Input: part model. Units: mm. Frame: model coordinates. A direction names the side the tool comes from. Coordinates: 2 decimals unless noted, no trailing zeros. Order: outer loops, then holes, each group sorted by start corner. A loop starts at its lowest first (then second) coordinate and runs counter-clockwise, first axis right, second up. Notation, with made-up numbers: M 1,-3.75 L 49,-3.75 A32 cw 49,25.25 Z; hole C 11.25,-39 d10. An arc over 180 degrees is marked long. Answer in a Markdown table with one row per item.
from build123d import *

# Parameters (mm, degrees)
SKETCH1_R                    = 4.25
BASE_FLANGE1_DEPTH           = 3.175
EDGE_FLANGE1_DEPTH           = 20
EDGE_FLANGE1_START           = 3.175
EDGE_FLANGE1_FLAT_DEPTH      = 3.175
EDGE_FLANGE3_STRIP_W         = 15.24
EDGE_FLANGE3_STRIP_H         = 3.175
EDGE_FLANGE3_STRIP_CUT_DEPTH = 20
EDGE_FLANGE3_DEPTH           = 20
EDGE_FLANGE3_START           = -3.175
EDGE_FLANGE3_PROFILE_R       = 4.25
EDGE_FLANGE3_FLAT_DEPTH      = 3.175


# Sheet-metal steps are written as plain solids
with BuildPart() as part:
    # Sketch1 → Base-Flange1 (new body)
    with BuildSketch(Plane.XY):
        with BuildLine():
            Line((12.5, 10), (0, 10))
            ThreePointArc((0, 10), (-10, 0), (0, -10))
            Line((0, -10), (12.5, -10))
            Line((12.5, -10), (12.5, 10))
        make_face()
        Circle(SKETCH1_R, mode=Mode.SUBTRACT)
    extrude(amount=-BASE_FLANGE1_DEPTH)

    # Edge-Flange1 bend section (across the edge) → Edge-Flange1 (add)
    with BuildSketch(Plane(origin=(13.77, -10, 0), x_dir=(-1, 0, 0), z_dir=(0, 1, 0))):
        with BuildLine():
            Line((-3.175, 1.27), (0, 1.27))
            ThreePointArc((0, 1.27), (0.371974388, 0.371974388), (1.27, 0))
            Line((1.27, 0), (1.27, -3.175))
            ThreePointArc((1.27, -3.175), (-1.873089642, -1.873089642), (-3.175, 1.27))
        make_face()
    extrude(amount=EDGE_FLANGE1_DEPTH)

    # Edge-Flange1 profile (on flange) → Edge-Flange1 flat (add)
    with BuildSketch(Plane.YZ.offset(13.77).offset(EDGE_FLANGE1_START)):
        with BuildLine():
            Line((36.2752, 26.825), (5, 26.825))
            ThreePointArc((5, 26.825), (-5.606601718, 22.431601718), (-10, 11.825))
            Line((-10, 11.825), (-10, 1.27))
            Line((-10, 1.27), (10, 1.27))
            Line((10, 1.27), (10, 1.825))
            ThreePointArc((10, 1.825), (11.464466094, 5.360533906), (15, 6.825))
            Line((15, 6.825), (36.2752, 6.825))
            Line((36.2752, 6.825), (36.2752, 26.825))
        make_face()
    extrude(amount=-EDGE_FLANGE1_FLAT_DEPTH)

    # Edge-Flange3 strip (across the edge) → Edge-Flange3 strip cut (cut)
    with BuildSketch(Plane(origin=(16.945, 36.2752, 6.825), x_dir=(0, -1, 0), z_dir=(0, 0, 1))):
        with Locations((-6.35, -1.5875)):
            Rectangle(EDGE_FLANGE3_STRIP_W, EDGE_FLANGE3_STRIP_H)
    extrude(amount=EDGE_FLANGE3_STRIP_CUT_DEPTH, mode=Mode.SUBTRACT)

    # Edge-Flange3 bend section (across the edge) → Edge-Flange3 (add)
    with BuildSketch(Plane(origin=(16.945, 36.2752, 6.825), x_dir=(0, -1, 0), z_dir=(0, 0, 1))):
        with BuildLine():
            Line((-3.175, 1.27), (0, 1.27))
            ThreePointArc((0, 1.27), (0.371974388, 0.371974388), (1.27, 0))
            Line((1.27, 0), (1.27, -3.175))
            ThreePointArc((1.27, -3.175), (-1.873089642, -1.873089642), (-3.175, 1.27))
        make_face()
    extrude(amount=EDGE_FLANGE3_DEPTH)

    # Edge-Flange3 profile (on flange) → Edge-Flange3 flat (add)
    with BuildSketch(Plane(origin=(16.945, 36.2752, 0), x_dir=(0, 0, -1), z_dir=(0, -1, 0)).offset(EDGE_FLANGE3_START)):
        with BuildLine():
            ThreePointArc((-6.825, 3.0675), (-14.14733047, 20.74516953), (-31.825, 28.0675))
            Line((-31.825, 28.0675), (-70.925400974, 28.0675))
            ThreePointArc((-70.925400974, 28.0675), (-79.925400974, 19.0675), (-70.925400974, 10.0675))
            Line((-70.925400974, 10.0675), (-31.825, 10.0675))
            ThreePointArc((-31.825, 10.0675), (-28.289466094, 8.603033906), (-26.825, 5.0675))
            Line((-26.825, 5.0675), (-26.825, 1.27))
            Line((-26.825, 1.27), (-6.825, 1.27))
            Line((-6.825, 1.27), (-6.825, 3.0675))
        make_face()
        with Locations((-70.925400974, 19.0675)):
            Circle(EDGE_FLANGE3_PROFILE_R, mode=Mode.SUBTRACT)
    extrude(amount=EDGE_FLANGE3_FLAT_DEPTH)


solid = part.part
1) Reachability of faces 1 (the face through (15, 27, 6.825)), 2 (the face through (35, 36.275, 44)), 3 (the face through (36.21, 37.885, 79.923)), 4 (the face through (13.77, 12, 14)) from +Z, -Z, +X, -X, +Y, -Y: full face, straight path, thin tool, end or side. Return the list, or none.
Resolved:
| item | result |
|---|---|
| face 1 | -Z, +X, -X, +Y |
| face 2 | +Z, -Z, +X, -Y |
| face 3 | +Z, +Y, -Y |
| face 4 | +Z, -X, +Y, -Y |
2) Material intervals for probe 1 along Y at (x, z) = (0, -1.7); probe 2 along Z at (x, y) = (6, 7.5) (3 decimals); probe 3 along X at (y, z) = (3, 11) (3 decimals), sorted ascending.
Resolved:
| item | result |
|---|---|
| probe 1 | y = -10 to -4.25, 4.25 to 10 |
| probe 2 | z = -3.175 to 0 |
| probe 3 | x = 13.77 to 16.945 |
3) Contact query for flat-ended pins moving along their axis: pin 1 (13.5 mm diameter, centred on x = 36.01, z = 70.93, fed in from -Y); pin 2 (1 mm diameter, centred on x = 16, y = 20.5, fed in from -Z) (3 decimals); pin 3 (3 mm diameter, centred on x = 12, z = 10, fed in from -Y); pin 4 (16 mm diameter, centred on x = 3, y = 1.5, fed in from +Z). Output: stop coordinate, or through.
Resolved:
| item | result |
|---|---|
| pin 1 | stops at y = 36.28 |
| pin 2 | stops at z = 6.825 |
| pin 3 | passes through |
| pin 4 | stops at z = 0 |
4) Cut plane D-D, the plane y = 17. Output: boundary loops of the cut face in (x, z) (3 decimals), and give its area (3 significant figures).
Resolved:
| item | result |
|---|---|
| outline | M 13.77,6.825 L 16.945,6.825 L 16.945,26.825 L 13.77,26.825 Z |
| area | 63.5 mm2 |
5) Cut plane B-B, the plane y = 0. Output: boundary loops of the cut face in (x, z) (3 decimals), and give its area (3 significant figures).
Resolved:
| item | result |
|---|---|
| outline | M -10,-3.175 L -4.25,-3.175 L -4.25,0 L -10,0 Z; M 4.25,-3.175 L 12.5,-3.175 A4.445 ccw 16.945,1.27 L 16.945,25.967 L 13.77,25.967 L 13.77,1.27 A1.27 cw 12.5,0 L 4.25,0 Z |
| area | 137 mm2 |
6) Mould query, pull axis X, two halves, no side actions, for faces 5 (the face through (9, 10, -1)), 6 (the face through (2.285, 3.584, -1.565)), 7 (the face through (-10, 0, -2)). Classes: +X half, -X half, draft (parallel to the pull), parting line (faces both ways), or undercut.
Resolved:
| item | result |
|---|---|
| face 5 | draft |
| face 6 | undercut |
| face 7 | -X half |
7) Cut plane A-A, the plane z = 74. Output: boundary loops of the cut face in (x, y).
Resolved:
| item | result |
|---|---|
| outline | M 27.55,36.28 L 33.08,36.28 L 33.08,39.45 L 27.55,39.45 Z; M 38.95,36.28 L 44.47,36.28 L 44.47,39.45 L 38.95,39.45 Z |
8) Cut plane C-C, the plane x = 5.5. Output: boundary loops of the cut face in (y, z) (3 decimals).
Resolved:
| item | result |
|---|---|
| outline | M -10,-3.175 L 10,-3.175 L 10,0 L -10,0 Z |
